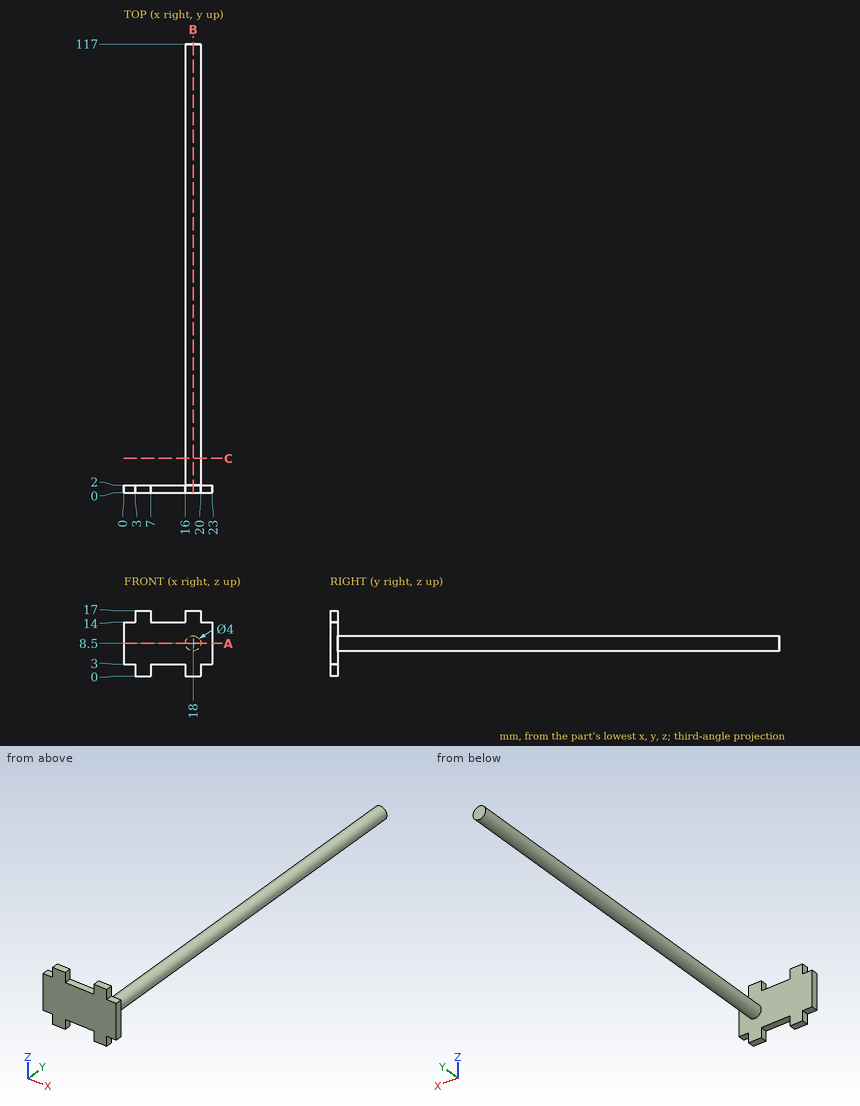
Job drawing, mm, ordinate dimensions from the low corner. One solid piece. Round coordinates to 2 decimals unless told otherwise and drop trailing zeros. Loops run counter-clockwise (first coordinate to the right, second up) from the corner with the lowest first, then second, coordinate; pieces in that order, holes last. Notation, with made-up numbers: (38, 41) -> (46, 41) arc R21 ccw to (46, 54) -> close; hole circle Ø5 at (38.5, -31). An arc over 180 degrees is marked (long way). One line per item, written item: value. Start each with the question number.
Q1. Cut at B-B on x = 18. List the corners of the cut face in (y, z).
Q2. Drop flat-ended pins along their axis: pin 1 Ø1 at (y, z) = (1.5, 15.5) entering from +X; pin 2 Ø4 at (y, z) = (37, 11.5) entering from +X; pin 3 Ø4 at (x, z) = (2.5, 14.5) entering from +Y; pin 4 Ø4 at (x, z) = (19.5, 5) entering from -Y. Give the stop position or say it passes through.
Q3. Cut at A-A on z = 8.5. List the corners of the cut face in (x, y).
Q4. Probe line 1 along X through (y, z) = (94, 8.25); line 2 along Y through (x, z) = (17, 1.5); line 3 along Z through (x, y) = (18.5, 68). List the from-to ranges inside material, lowest first.
Q5. Cut at C-C on y = 9. List the corners of the cut face in (x, z).
Computed:
1. outline: (0, 0) -> (2, 0) -> (2, 6.5) -> (117, 6.5) -> (117, 10.5) -> (2, 10.5) -> (2, 17) -> (0, 17) -> close
2. pin 1: x = 20
2. pin 2: x = 19.73
2. pin 3: y = 2
2. pin 4: y = 0
3. outline: (0, 0) -> (23, 0) -> (23, 2) -> (20, 2) -> (20, 117) -> (16, 117) -> (16, 2) -> (0, 2) -> close
4. line 1: 16.02 to 19.98
4. line 2: 0 to 2
4. line 3: 6.56 to 10.44
5. outline: circle Ø4 at (18, 8.5)
